Input: dimensioned drawing with shaded views. Units: mm. Origin: part minimum x, y, z. A direction names the side the tool comes from. Round coordinates to 2 decimals unless told otherwise and drop trailing zeros. Order: outer loops, then holes, each group sorted by start corner. A loop starts at its lowest first (then second) coordinate and runs counter-clockwise, first axis right, second up. Notation, with made-up numbers: (47, 9) - (74, 9) arc R18 ccw to (74, 14) - close; hole circle Ø11 at (83, -17.75). An arc over 180 degrees is marked (long way). Put each result on its own line as item: value. Start each with the question number.
(1) Pull-direction query (X, two-part tool) for the marked faces 1, 2, 3 and 4; classes: released by +X, released by -X, zero draft, split by the parting line, or undercut.
(2) Access query for the marked faces 5, 6, 7, 8 and 9. Directions: +Z, -Z, +X, -X, +Y, -Y. A direction counts if a zero-diameter tool reaches every point of the face in a straight line with its end or side. Return the directions, or none.
(3) Material intervals for L1, parallel to Z at x = 26, y = 13; L2, parallel to X at y = 5.5, z = 8; L3, parallel to X at y = 17.5, z = 3.5, sorted ascending. Write a range as [from, to].
(4) Pin query (flat end, axial travel): P1, Ø4, axis at y = 38, z = 16.5, coming from the -X side; P2, Ø16.5, axis at y = 24.5, z = 11, coming from the +X side; P3, Ø12.5, axis at x = 21.5, z = 37.5, coming from the -Y side; P4, Ø8, axis at x = 34.5, z = 38, coming from the +Y side. Return the tip coordinate at first contact, or that it passes through.
(5) Section D-D (y = 9). Output: boundary loops of the cut face in (x, z), and give its area (3 significant figures).
(6) Section B-B (x = 20.5). Output: boundary loops of the cut face in (y, z).
(7) Section C-C (z = 21). Output: boundary loops of the cut face in (x, y).
(8) Section A-A (x = 37.5). Output: boundary loops of the cut face in (y, z).
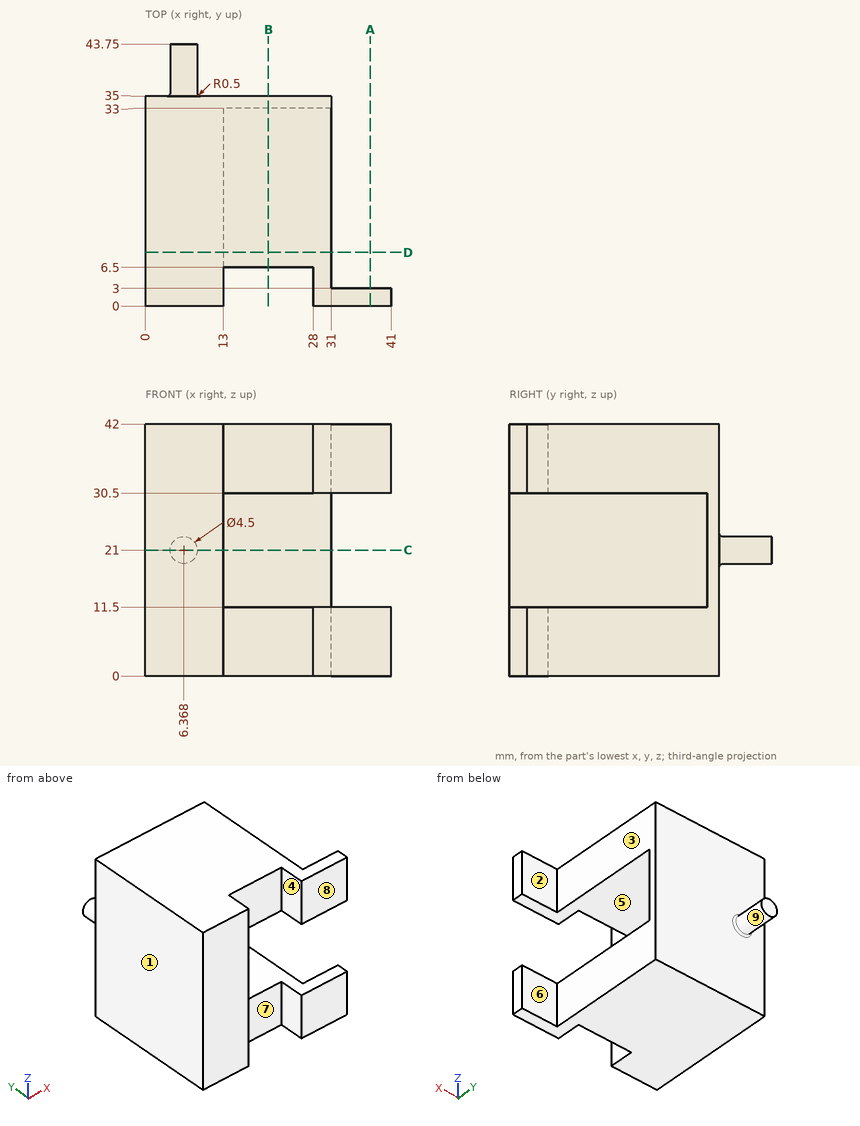
Checks:
1. face 1: released by -X
1. face 2: zero draft
1. face 3: released by +X
1. face 4: undercut
2. face 5: +X, -Y
2. face 6: +Z, -Z, +X, +Y
2. face 7: +Z, -Z, -Y
2. face 8: +Z, -Z, +X, -X, -Y
2. face 9: +Y
3. L1: z = [0, 11.5], [30.5, 42]
3. L2: x = [0, 13], [28, 31]
3. L3: x = [0, 31]
4. P1: passes through
4. P2: stops at x = 31
4. P3: stops at y = 6.5
4. P4: stops at y = 35
5. outline: (0, 0) - (31, 0) - (31, 11.5) - (13, 11.5) - (13, 30.5) - (31, 30.5) - (31, 42) - (0, 42) - close
5. area: 960 mm²
6. outline: (6.5, 0) - (35, 0) - (35, 42) - (6.5, 42) - (6.5, 30.5) - (33, 30.5) - (33, 11.5) - (6.5, 11.5) - close
7. outline: (0, 0) - (13, 0) - (13, 33) - (31, 33) - (31, 35) - (9.12, 35) arc R0.5 cw to (8.62, 35.5) - (8.62, 43.75) - (4.12, 43.75) - (4.12, 35.5) arc R0.5 cw to (3.62, 35) - (0, 35) - close
8. outline: (0, 0) - (3, 0) - (3, 11.5) - (0, 11.5) - close; (0, 30.5) - (3, 30.5) - (3, 42) - (0, 42) - close
